Build history of the part. All positions in model axes, mm. Face numbers are marked on the shaded views. A direction names the side the tool comes from. Round coordinates to 2 decimals unless told otherwise and drop trailing zeros. Order: outer loops, then holes, each group sorted by start corner. A loop starts at its lowest first (then second) coordinate and runs counter-clockwise, first axis right, second up. Notation, with made-up numbers: (38, 69.25) -> (61, 69.25) arc R7 cw to (61, 81.25) -> close; hole circle Ø11 at (-37.75, -21.75). An arc over 180 degrees is marked (long way). Answer as a JSON object with one key per item and string values.
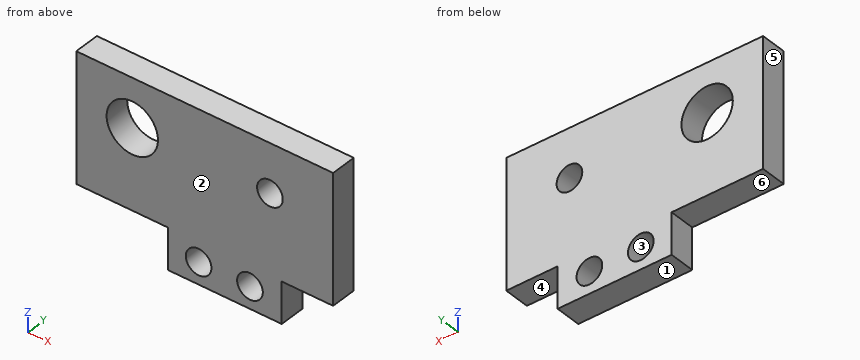
from build123d import *

# Parameters (mm, degrees)
F0_W     = 63.5
F0_H     = 12.7
F0_W_2   = 28.1816057964
F0_H_2   = 5.08
F1_DEPTH = 6.35
F2_D     = 12.7
F2_DEPTH = 12.7
F2_TIP   = 3.8154649308
F3_D     = 6.35
F3_DEPTH = 12.7
F3_TIP   = 1.9077324654
F4_D     = 6.35
F4_DEPTH = 12.7
F4_TIP   = 1.9077324654


with BuildPart() as f1:
    # F0 (on Front) → F1 (new body)
    with BuildSketch(Plane.XZ):
        with Locations((8.7264817292, 15.5304455166)):
            Rectangle(F0_W, F0_H)
        Polygon((40.4764817292, 9.1804455166), (-23.0235182708, 9.1804455166), (-23.0235182708, -9.8695544834), (-0.4051240673, -9.8695544834), (-0.4051240673, -14.9495544834), (27.7764817292, -14.9495544834), (27.7764817292, -9.8695544834), (40.4764817292, -9.8695544834), align=None)
        with Locations((13.685678831, -17.4895544834)):
            Rectangle(F0_W_2, F0_H_2)
    extrude(amount=F1_DEPTH)

    # F2
    with Locations(Plane(origin=(0, 0, 0), x_dir=(1, 0, 0), z_dir=(0, 1, 0))):
        with Locations((-9.1782798991, -9.8773387097)):
            Hole(F2_D / 2, depth=F2_DEPTH)
            with Locations((0, 0, -(F2_DEPTH + F2_TIP / 2))):  # 118° drill point
                Cone(0, F2_D / 2, F2_TIP, mode=Mode.SUBTRACT)

    # F3
    with Locations(Plane(origin=(0, 0, 0), x_dir=(1, 0, 0), z_dir=(0, 1, 0))):
        with Locations((24.8577201009, -9.8773387097)):
            Hole(F3_D / 2, depth=F3_DEPTH)
            with Locations((0, 0, -(F3_DEPTH + F3_TIP / 2))):  # 118° drill point
                Cone(0, F3_D / 2, F3_TIP, mode=Mode.SUBTRACT)

    # F4
    with Locations(Plane(origin=(0, 0, 0), x_dir=(1, 0, 0), z_dir=(0, 1, 0))):
        with Locations((7.2235863984, 14.6380947129), (19.9235863984, 14.6380947129)):
            Hole(F4_D / 2, depth=F4_DEPTH)
            with Locations((0, 0, -(F4_DEPTH + F4_TIP / 2))):  # 118° drill point
                Cone(0, F4_D / 2, F4_TIP, mode=Mode.SUBTRACT)


solid = f1.part
1) Flat gauge pins, fed straight in: pin 1 Ø1.9 at (x, y) = (37, -2) entering from -Z; pin 2 Ø10 at (x, z) = (7.22, -14.64) entering from -Y; pin 3 Ø3 at (y, z) = (-2, -13.5) entering from +X. Where does each tip first touch, or does it go through?
Checked values:
{"pin 1": "stops at z = -9.87", "pin 2": "stops at y = -6.35", "pin 3": "stops at x = 27.78"}
2) Cut at B-B, the plane z = 4.5. Give the cut face in (x, y).
Checked values:
{"outline": "(-23.02, -6.35) -> (-12.56, -6.35) -> (-12.56, 0) -> (-23.02, 0) -> close; (-5.8, -6.35) -> (40.48, -6.35) -> (40.48, 0) -> (-5.8, 0) -> close"}
3) Cut at A-A, the plane x = 21. Give the cut face in (y, z), plus the area to 3 significant figures.
Checked values:
{"outline": "(-6.35, -20.03) -> (0, -20.03) -> (0, -17.63) -> (-6.35, -17.63) -> close; (-6.35, -11.65) -> (0, -11.65) -> (0, 21.88) -> (-6.35, 21.88) -> close", "area": "228 mm²"}
4) Probe L1, parallel to X at y = -1.75, z = -14.5; L2, parallel to X at y = -1.75, z = -16; L3, parallel to Z at x = 7, y = -3.75. List the from-to ranges inside material, lowest first. Write a range as from..to.
Checked values:
{"L1": "x = -0.41..4.05, 10.4..16.75, 23.1..27.78", "L2": "x = -0.41..4.36, 10.09..17.06, 22.79..27.78", "L3": "z = -20.03..-17.81, -11.47..21.88"}
5) Which spindle directions (+Z, -Z, +X, -X, +Y, -Y) get a long thin tool onto all of the face, cutting with end or side? Do the marked faces 4, 5 and 6. Say none if no direction does.
Checked values:
{"face 4": "-Z, +X, +Y, -Y", "face 5": "+Z, -Z, -X, +Y, -Y", "face 6": "-Z, -X, +Y, -Y"}
6) Cut at C-C, the plane y = -2. Give the cut face in (x, z) (3 decimals).
Checked values:
{"outline": "(-23.024, -9.87) -> (-0.405, -9.87) -> (-0.405, -20.03) -> (27.776, -20.03) -> (27.776, -9.87) -> (40.476, -9.87) -> (40.476, 21.88) -> (-23.024, 21.88) -> close; hole circle Ø12.7 at (-9.178, 9.877); hole circle Ø6.35 at (7.224, -14.638); hole circle Ø6.35 at (19.924, -14.638); hole circle Ø6.35 at (24.858, 9.877)"}
7) Pull direction Z, two halves, no side cores. Call the marked faces 1, 2 and 3: pulls with the +Z half, pulls with the -Z half, needs draft (parallel to the pull), parting line crosses it, or undercut.
Checked values:
{"face 1": "pulls with the -Z half", "face 2": "needs draft", "face 3": "undercut"}
8) Cut at D-D, the plane z = -10.5. Give the cut face in (x, y).
Checked values:
{"outline": "(-0.41, -6.35) -> (27.78, -6.35) -> (27.78, 0) -> (-0.41, 0) -> close"}
